Could you check a few things on this drawing? It's one solid part, dimensions in mm from its lowest x, y, z. Give positions to 0.01 mm unless a question says otherwise; leave off trailing zeros. Order: outer loops, then holes, each group sorted by start corner. A loop starts at its lowest first (then second) coordinate and runs counter-clockwise, first axis right, second up.
Item 1: I'm going to push flat-ended pins straight in: pin 1 Ø5 at (x, y) = (21.5, 29) entering from -Z; pin 2 Ø8.5 at (x, y) = (98.5, 10) entering from -Z. Where does each tip first touch, or does it pass through?
Item 2: If I drill on line 1 along Y through (x, z) = (98.5, 1.15); line 2 along X through (y, z) = (28.4, 0.85); line 3 along X through (y, z) = (44, 0.8), over which ranges is the centre line in solid material (lowest first)?
Item 3: I want a section at B-B, the plane y = 10. Write out the boundary of the cut face in (x, z).
Item 4: I want a section at C-C, the plane x = 21.8. Write out the boundary of the cut face in (y, z).
Item 5: I want a section at A-A, the plane x = 98.5. Write out the boundary of the cut face in (y, z).
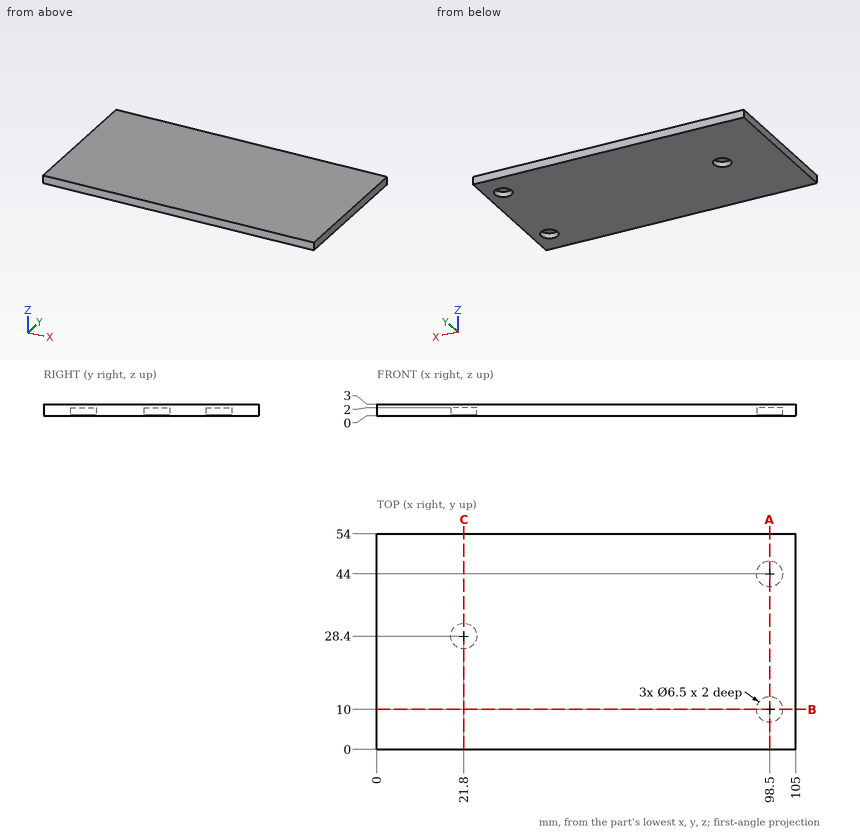
Results list:
1. pin 1: stops at z = 2
1. pin 2: stops at z = 0
2. line 1: y = 0 to 6.75, 13.25 to 40.75, 47.25 to 54
2. line 2: x = 0 to 18.55, 25.05 to 105
2. line 3: x = 0 to 95.25, 101.75 to 105
3. outline: (0, 0) - (95.25, 0) - (95.25, 2) - (101.75, 2) - (101.75, 0) - (105, 0) - (105, 3) - (0, 3) - close
4. outline: (0, 0) - (25.15, 0) - (25.15, 2) - (31.65, 2) - (31.65, 0) - (54, 0) - (54, 3) - (0, 3) - close
5. outline: (0, 0) - (6.75, 0) - (6.75, 2) - (13.25, 2) - (13.25, 0) - (40.75, 0) - (40.75, 2) - (47.25, 2) - (47.25, 0) - (54, 0) - (54, 3) - (0, 3) - close
